Build history of the part. All positions in model axes, mm. Face numbers are marked on the shaded views. A direction names the side the tool comes from. Round coordinates to 2 decimals unless told otherwise and drop trailing zeros. Order: outer loops, then holes, each group sorted by start corner. A loop starts at its lowest first (then second) coordinate and runs counter-clockwise, first axis right, second up. Notation, with made-up numbers: (-26.5, 73.5) -> (13.5, 73.5) arc R15 cw to (13.5, 101.5) -> close; hole circle Ø5 at (11.25, -13). An arc over 180 degrees is marked (long way). Answer as a JSON object with one key per item and string values.
Autodesk Inventor part; units mm, degrees
ref_plane "YZ Plane" through (0, 0, 0) normal (1, 0, 0) x (0, 1, 0)
ref_plane "XZ Plane" through (0, 0, 0) normal (0, 1, 0) x (-1, 0, 0)
ref_plane "XY Plane" through (0, 0, 0) normal (0, 0, 1) x (1, 0, 0)
sketch "Skizze1" plane through (0, 0, 0) normal (1, 0, 0) x (0, 1, 0)
  line L0 (3, 8.0893) -> (5.1212, 8.0893) construction
  line L1 (-0.0509, -6) -> (0.0741, -6) construction
  line L2 (0.0741, -6) -> (0.0741, 6) construction
  line L3 (0.0741, 6) -> (-0.0509, 6) construction
  line L4 (-0.0509, 6) -> (-0.0509, -6) construction
  line L5 (-0.0509, -6) -> (0.0741, 6) construction
  line L6 (0.0741, -6) -> (-0.0509, 6) construction
  line L7 (-0.0509, 6) -> (-0.0509, 0)
  line L8 (-0.0509, 0) -> (-0.3509, 0)
  line L9 (-0.3509, 0) -> (-0.3509, 6.7569)
  line L10 (-0.3509, 6.7569) -> (0.8491, 7.9569)
  line L11 (0.8491, 7.9569) -> (0.8491, 8.3023)
  line L12 (-0.0509, 6) -> (-0.0509, 6.2)
  line L13 (-0.0509, 6.2) -> (1.4491, 7.7)
  line L14 (1.4491, 7.7) -> (1.4491, 8.5508)
  line L15 (1.4491, 8.5508) -> (-0.7509, 10.7508)
  line L16 (-1.3509, 12.5) -> (-1.3509, 9.3023)
  line L17 (0.8491, 8.3023) -> (-0.1509, 9.3023)
  line L18 (-0.1509, 9.3023) -> (-1.3509, 9.3023)
  line L19 (-0.7509, 10.7508) -> (-0.7509, 12.5)
  line L20 (-0.7509, 12.5) -> (-1.3509, 12.5)
  point P0 (0.0116, 0)
  point P1 (0.0116, 0)
  dimension "d14" = 0.125
  dimension "d15" = 12
  dimension "d16" = 0.3
  dimension "d18" = 135
  dimension "d20" = 0.2
  dimension "d27" = 135
  dimension "d28" = 1
  dimension "d29" = 1.2
  dimension "d30" = 0.6
  dimension "d31" = 0.6
  dimension "d34" = 1
  dimension "d36" = 0.6
  dimension "d37" = 12.5
revolve "Umdrehung1" add sketch "Skizze1" angle 360 about axis through (0, -0.0509, 0) along (0, -1, 0)
properties part number "50_ETL_Membrane_v0"
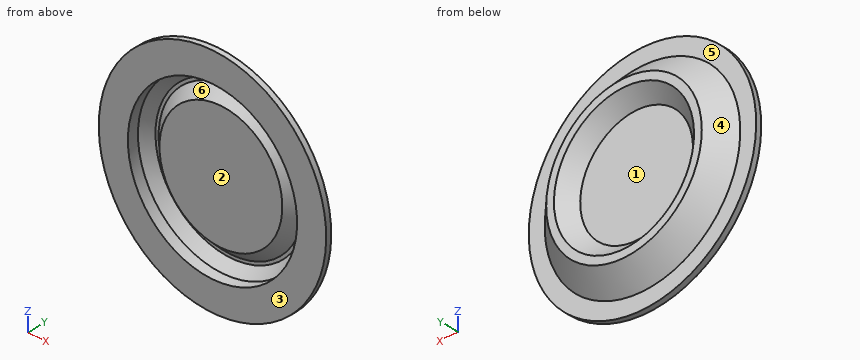
1) Which spindle directions (+Z, -Z, +X, -X, +Y, -Y) get a long thin tool onto all of the face, cutting with end or side? Do the marked faces 1, 2 and 3. Say none if no direction does.
Checked values:
{"face 1": "+Y", "face 2": "-Y", "face 3": "+Z, -Z, +X, -X, -Y"}
2) Probe L1, parallel to X at y = -0.8, z = 0; L2, parallel to Z at x = -4.5, y = -0.25. List the from-to ranges inside material, lowest first. Write a range as from..to.
Checked values:
{"L1": "x = -12.5..-9.3, 9.3..12.5", "L2": "z = -9.21..-8.14, -5.17..5.17, 8.14..9.21"}
3) Pull direction X, two halves, no side cores. Call the marked faces 4, 5 and 6: pulls with the +X half, pulls with the -X half, needs draft (parallel to the pull), parting line crosses it, or undercut.
Checked values:
{"face 4": "parting line crosses it", "face 5": "needs draft", "face 6": "undercut"}
4) Cut at B-B, the plane x = 0. Give the cut face in (y, z), plus the area to 3 significant figures.
Checked values:
{"outline": "(-1.35, -12.5) -> (-0.75, -12.5) -> (-0.75, -10.75) -> (1.45, -8.55) -> (1.45, -7.7) -> (-0.05, -6.2) -> (-0.05, 6.2) -> (1.45, 7.7) -> (1.45, 8.55) -> (-0.75, 10.75) -> (-0.75, 12.5) -> (-1.35, 12.5) -> (-1.35, 9.3) -> (-0.15, 9.3) -> (0.85, 8.3) -> (0.85, 7.96) -> (-0.35, 6.76) -> (-0.35, -6.76) -> (0.85, -7.96) -> (0.85, -8.3) -> (-0.15, -9.3) -> (-1.35, -9.3) -> close", "area": "14.3 mm²"}
5) Flat gauge pins, fed straight in: pin 1 Ø4 at (x, z) = (-2.5, 2.5) entering from -Y; pin 2 Ø13.5 at (x, z) = (2, 1) entering from +Y; pin 3 Ø4 at (x, z) = (-9.5, -5.5) entering from +Y; pin 4 Ø1 at (x, y) = (8, -1) entering from -Z. Where does each tip first touch, or does it go through?
Checked values:
{"pin 1": "stops at y = -0.35", "pin 2": "stops at y = 1.45", "pin 3": "stops at y = 1.02", "pin 4": "stops at z = -10"}
6) Cut at A-A, the plane z = 0. Give the cut face in (x, y).
Checked values:
{"outline": "(-12.5, -1.35) -> (-9.3, -1.35) -> (-9.3, -0.15) -> (-8.3, 0.85) -> (-7.96, 0.85) -> (-6.76, -0.35) -> (6.76, -0.35) -> (7.96, 0.85) -> (8.3, 0.85) -> (9.3, -0.15) -> (9.3, -1.35) -> (12.5, -1.35) -> (12.5, -0.75) -> (10.75, -0.75) -> (8.55, 1.45) -> (7.7, 1.45) -> (6.2, -0.05) -> (-6.2, -0.05) -> (-7.7, 1.45) -> (-8.55, 1.45) -> (-10.75, -0.75) -> (-12.5, -0.75) -> close"}
7) Cut at C-C, the plane y = 0.55. Give the cut face in (x, z).
Checked values:
{"outline": "circle Ø18.9 at (0, 0); circle Ø15.32 at (0, 0); hole circle Ø17.2 at (0, 0); hole circle Ø13.6 at (0, 0)"}
